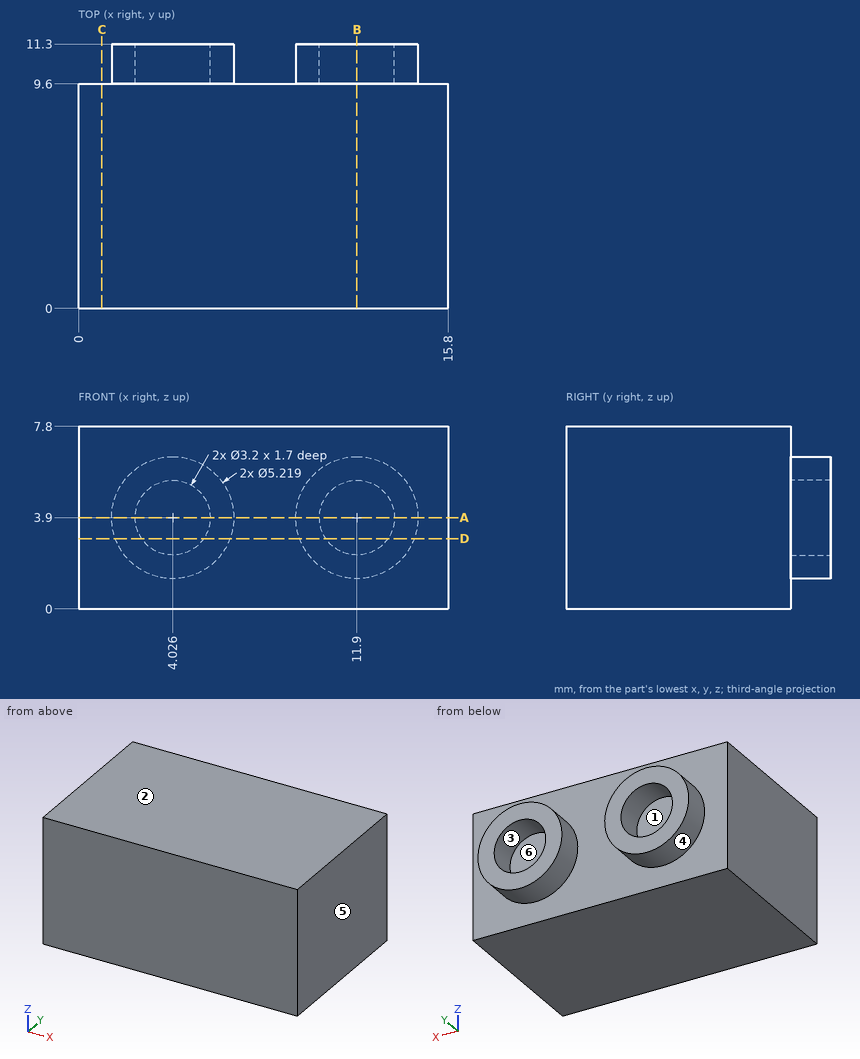
Source: three-view drawing plus pictorial views. Frame: mm from the lowest corner of the part. A direction names the side the tool comes from. Coordinates: 2 decimals unless noted, no trailing zeros. Loops run counter-clockwise (first coordinate to the right, second up) from the corner with the lowest first, then second, coordinate; pieces in that order, holes last. Notation, with made-up numbers: (78, 66) -> (92, 66) arc R18 ccw to (92, 89) -> close; hole circle Ø2 at (64, 66). An arc over 180 degrees is marked (long way). Write each question's results on one line, items separated by ' | '. Start each with the question number.
Q1. Reachability of the marked faces 1 and 2 from +Z, -Z, +X, -X, +Y, -Y: full face, straight path, thin tool, end or side. Return the list, or none.
Q2. Section A-A, the plane z = 3.9. Return the cut outline in (x, y) (1 decimal), plus the area to 3 significant figures.
Q3. Section C-C, the plane x = 1. Return the cut outline in (y, z).
Q4. Section D-D, the plane z = 3. Return the cut outline in (x, y) (1 decimal).
Q5. Pull-direction query (Z, two-part tool) for the marked faces 3, 4, 5 and 6; classes: released by +Z, released by -Z, zero draft, split by the parting line, or undercut.
Q6. Pin query (flat end, axial travel): pin 1 (1 mm diameter, centred on x = 12, z = 4, fed in from +Y). Return the tip coordinate at first contact, or that it passes through.
Q7. Ray query, line 1 (X direction, y = 10.45, z = 3.9) (1 decimal); line 2 (Y direction, x = 4.25, z = 7.75). Return the intervals inside material, ascending. Write a range as from..to.
Q8. Section B-B, the plane x = 11.9. Return the cut outline in (y, z).
Found:
1) face 1: +Y | face 2: +Z, +X, -X, +Y, -Y
2) outline: (0, 0) -> (15.8, 0) -> (15.8, 9.6) -> (14.5, 9.6) -> (14.5, 11.3) -> (13.5, 11.3) -> (13.5, 9.6) -> (10.3, 9.6) -> (10.3, 11.3) -> (9.3, 11.3) -> (9.3, 9.6) -> (6.6, 9.6) -> (6.6, 11.3) -> (5.6, 11.3) -> (5.6, 9.6) -> (2.4, 9.6) -> (2.4, 11.3) -> (1.4, 11.3) -> (1.4, 9.6) -> (0, 9.6) -> close | area: 159 mm2
3) outline: (0, 0) -> (9.6, 0) -> (9.6, 7.8) -> (0, 7.8) -> close
4) outline: (0, 0) -> (15.8, 0) -> (15.8, 9.6) -> (14.3, 9.6) -> (14.3, 11.3) -> (13.2, 11.3) -> (13.2, 9.6) -> (10.6, 9.6) -> (10.6, 11.3) -> (9.5, 11.3) -> (9.5, 9.6) -> (6.5, 9.6) -> (6.5, 11.3) -> (5.3, 11.3) -> (5.3, 9.6) -> (2.7, 9.6) -> (2.7, 11.3) -> (1.6, 11.3) -> (1.6, 9.6) -> (0, 9.6) -> close
5) face 3: undercut | face 4: split by the parting line | face 5: zero draft | face 6: undercut
6) pin 1: y = 9.6
7) line 1: 1.4..2.4, 5.6..6.6, 9.3..10.3, 13.5..14.5 | line 2: 0..9.6
8) outline: (0, 0) -> (9.6, 0) -> (9.6, 1.29) -> (11.3, 1.29) -> (11.3, 2.3) -> (9.6, 2.3) -> (9.6, 5.5) -> (11.3, 5.5) -> (11.3, 6.51) -> (9.6, 6.51) -> (9.6, 7.8) -> (0, 7.8) -> close
